Part model, mm, in its own coordinate system. A direction names the side the tool comes from. Round coordinates to 2 decimals unless told otherwise and drop trailing zeros. Loops run counter-clockwise (first coordinate to the right, second up) from the corner with the lowest first, then second, coordinate; pieces in that order, holes last. Notation, with made-up numbers: M 50.25,1 L 65.25,1 A19 cw 65.25,16 Z; hole C 89,-24.75 d9. An arc over 180 degrees is marked long. Answer as CSV lines item,"result". Start each with the question number.
Item 1: Mould opens along X. For faces 1 (the cylindrical face through (30.911, 1.14, 40.313)), 2 (the flat face through (44, 3.492, 0)), 3 (the cylindrical face through (-12.894, 2.798, -40.944)) say: pulls with the +X half, pulls with the -X half, needs draft (parallel to the pull), parting line crosses it, or undercut.
Item 2: Wall check: line 1 (X direction, y = 2.8, z = 0); line 2 (X direction, y = 2.6, z = 0); line 3 (X direction, y = 1.55, z = 0). Give the ranges that are in metal, low to high.
Item 3: Drop flat-ended pins along their axis: pin 1 Ø5 at (x, z) = (-9, 10) entering from -Y; pin 2 Ø10 at (x, z) = (4, 35) entering from -Y; pin 3 Ø1 at (x, z) = (35.5, 23) entering from +Y. Give the stop position or say it passes through.
Item 4: Band-saw the part on B-B (z = 0). Give the cut face in (x, y) (1 decimal), and give its area (3 significant figures).
Item 5: Which spindle directions (+Z, -Z, +X, -X, +Y, -Y) get a long thin tool onto all of the face, cutting with end or side? Do faces 4 (the flat face through (-32, 2.096, -22)), 5 (the flat face through (22, 0, 1)). Say none if no direction does.
Item 6: Band-saw the part on A-A (x = 0). Give the cut face in (y, z) (1 decimal), and give its area (3 significant figures).
```python
from build123d import *

# Parameters (mm, degrees)
FILLET1_R = 0.396875
FILLET2_R = 1.5875


with BuildPart() as part:
    # Sketch1 → Revolve1 (revolve)
    with BuildSketch(Plane.XY, mode=Mode.PRIVATE) as revolve1_sk:
        Polygon((17.526, 0), (17.526, 2.0955), (17.526, 4.7625), (38.1, 4.7625), (38.1, 2.0955), (42.926, 2.0955), (42.926, 3.4925), (50.8, 3.4925), (50.8, 0), align=None)
    revolve(revolve1_sk.sketch.rotate(Axis((0, 0, 0), (0, 1, 0)), 90), axis=Axis((0, 0, 0), (0, 1, 0)))

    # Fillet1
    fillet1_edges = [part.edges().sort_by_distance(p)[0] for p in [
        (0, 0, 50.8),
        (0, 3.4925, 42.926),
        (0, 2.0955, 42.926),
        (0, 2.0955, 38.1),
    ]]
    fillet(fillet1_edges, radius=FILLET1_R)

    # Fillet2
    fillet2_edges = [part.edges().sort_by_distance(p)[0] for p in [
        (0, 3.4925, 50.8),
    ]]
    fillet(fillet2_edges, radius=FILLET2_R)


solid = part.part
```
Answer block:
1,face 1,"parting line crosses it"
1,face 2,"needs draft"
1,face 3,"undercut"
2,line 1,"x = -50.52 to -42.93, -38.1 to -17.53, 17.53 to 38.1, 42.93 to 50.52"
2,line 2,"x = -50.64 to -42.93, -38.1 to -17.53, 17.53 to 38.1, 42.93 to 50.64"
2,line 3,"x = -50.8 to -17.53, 17.53 to 50.8"
3,pin 1,"passes through"
3,pin 2,"stops at y = 0"
3,pin 3,"stops at y = 2.2"
4,outline,"M -50.8,0.4 A0.4 ccw -50.4,0 L -17.5,0 L -17.5,4.8 L -38.1,4.8 L -38.1,2.5 A0.4 cw -38.5,2.1 L -42.5,2.1 A0.4 cw -42.9,2.5 L -42.9,3.1 A0.4 ccw -43.3,3.5 L -49.2,3.5 A1.6 ccw -50.8,1.9 Z; M 17.5,0 L 50.4,0 A0.4 ccw 50.8,0.4 L 50.8,1.9 A1.6 ccw 49.2,3.5 L 43.3,3.5 A0.4 ccw 42.9,3.1 L 42.9,2.5 A0.4 cw 42.5,2.1 L 38.5,2.1 A0.4 cw 38.1,2.5 L 38.1,4.8 L 17.5,4.8 Z"
4,area,"270 mm^2"
5,face 4,"+Y"
5,face 5,"+Z, -Z, +X, -X, -Y"
6,outline,"M 0,-50.4 A0.4 ccw 0.4,-50.8 L 1.9,-50.8 A1.6 ccw 3.5,-49.2 L 3.5,-43.3 A0.4 ccw 3.1,-42.9 L 2.5,-42.9 A0.4 cw 2.1,-42.5 L 2.1,-38.5 A0.4 cw 2.5,-38.1 L 4.8,-38.1 L 4.8,-17.5 L 0,-17.5 Z; M 0,17.5 L 4.8,17.5 L 4.8,38.1 L 2.5,38.1 A0.4 cw 2.1,38.5 L 2.1,42.5 A0.4 cw 2.5,42.9 L 3.1,42.9 A0.4 ccw 3.5,43.3 L 3.5,49.2 A1.6 ccw 1.9,50.8 L 0.4,50.8 A0.4 ccw 0,50.4 Z"
6,area,"270 mm^2"
